from build123d import *

# Parameters (mm, degrees)
SKETCH1_R           = 3
BOSS_EXTRUDE2_DEPTH = 10
FILLET1_R           = 20
FILLET2_R           = 20
CUT_EXTRUDE1_START  = -10
CUT_EXTRUDE1_DEPTH  = 10
FILLET3_R           = 5
CUT_EXTRUDE4_START  = -10
CUT_EXTRUDE4_DEPTH  = 10


with BuildPart() as part:
    # Sketch1 → Boss-Extrude2 (new body)
    with BuildSketch(Plane.XY):
        with BuildLine():
            Line((-30, 15.770412854), (-30, 0))
            Line((-30, 0), (-17.5, -210))
            ThreePointArc((-17.5, -210), (0, -227.5), (17.5, -210))
            Line((17.5, -210), (30, 0))
            Line((30, 0), (30, 15.770412854))
            Line((30, 15.770412854), (-30, 15.770412854))
        make_face()
        with Locations((-15, 0)):
            Circle(SKETCH1_R, mode=Mode.SUBTRACT)
        with Locations((15, 0)):
            Circle(SKETCH1_R, mode=Mode.SUBTRACT)
        Polygon((0, -205), (6, -205), (6, -215), (-6, -215), (-6, -205), align=None, mode=Mode.SUBTRACT)
    extrude(amount=BOSS_EXTRUDE2_DEPTH)

    # Fillet1
    fillet1_edges = [part.edges().sort_by_distance(p)[0] for p in [
        (-30, 15.770412854, 5),
    ]]
    fillet(fillet1_edges, radius=FILLET1_R)

    # Fillet2
    fillet2_edges = [part.edges().sort_by_distance(p)[0] for p in [
        (30, 15.770412854, 5),
    ]]
    fillet(fillet2_edges, radius=FILLET2_R)

    # Sketch4 → Cut-Extrude1 (cut)
    with BuildSketch(Plane.XY.offset(10).offset(CUT_EXTRUDE1_START)):
        Polygon((-15.651797422, -15), (0.190220551, -102.160979768), (15.643622882, -15), (15, -15), align=None)
        Polygon((-22.473027071, -25.6531452), (-13.367328465, -178.628881795), (-4.134156204, -126.551525408), align=None)
        Polygon((22.230419841, -27.161313899), (4.615986353, -126.511039477), (13.430162671, -175.005634359), align=None)
        with BuildLine():
            Line((0.291609598, -150.901585116), (-7.372445375, -194.128735111))
            ThreePointArc((-7.372445375, -194.128735111), (0.476576628, -192.506490497), (8.225632191, -194.553674383))
            Line((8.225632191, -194.553674383), (0.291609598, -150.901585116))
        make_face()
    extrude(amount=CUT_EXTRUDE1_DEPTH, mode=Mode.SUBTRACT)

    # Fillet3
    fillet3_edges = [part.edges().sort_by_distance(p)[0] for p in [
        (8.225632191, -194.553674383, 5),
        (-7.372445375, -194.128735111, 5),
        (-15.651797422, -15, 5),
        (15.643622882, -15, 5),
    ]]
    fillet(fillet3_edges, radius=FILLET3_R)

    # Sketch5 → Cut-Extrude4 (cut)
    with BuildSketch(Plane.XY.offset(10).offset(CUT_EXTRUDE4_START)):
        with BuildLine():
            Line((29.260488635, 0), (18, 0))
            ThreePointArc((18, 0), (17.738612788, -1.224744871), (17, -2.236067977))
            Line((17, -2.236067977), (17, -18))
            Line((17, -18), (28.928571429, -18))
            Line((28.928571429, -18), (29.677502384, -5.417959945))
            ThreePointArc((29.677502384, -5.417959945), (29.653859351, -2.694751229), (29.260488635, 0))
        make_face()
        with BuildLine():
            ThreePointArc((17, 2.236067977), (17.738612788, 1.224744871), (18, 0))
            Line((18, 0), (29.260488635, 0))
            ThreePointArc((29.260488635, 0), (24.938968919, 8.738256866), (17, 14.39559177))
            Line((17, 14.39559177), (17, 2.236067977))
        make_face()
    extrude(amount=CUT_EXTRUDE4_DEPTH, mode=Mode.SUBTRACT)


solid = part.part
Build history of the part. All positions in model axes, mm. A direction names the side the tool comes from. Coordinates: 2 decimals unless noted, no trailing zeros. Write each loop counter-clockwise with the first axis right and the second up, starting at its lowest first coordinate (ties: lowest second). Pieces come first, ordered by that corner, then holes.
(1) Cut at B-B on y = -71.5. List the corners of the cut face in (x, z), and give its area (3 significant figures).
(2) Cut at C-C on z = 4.5. State how many separate pieces and enclosed holes the cut face has, and give its area (3 significant figures).
(3) Mould opens along Y. For faces 1 (the flat face through (7.295, -62.086, 4.93)), 2 (the cylindrical face through (-0.385, -227.496, 4.93)), 3 (the flat face through (-1, -104, 10)) say: pulls with the +Y half, pulls with the -Y half, needs draft (parallel to the pull), parting line crosses it, or undercut.
(4) Drill centre lines: line 1 (X direction, y = -43.5, z = 3.75); line 2 (X direction, y = -173, z = 4.75); line 3 (X direction, y = -145, z = 2.5). Where is each one in solid material? Low to high.
(5) Pin check, flat tips, straight feed: pin 1 Ø5 at (y, z) = (-209, 5) entering from +X; pin 2 Ø2 at (y, z) = (-190.5, 4) entering from +X; pin 3 Ø1 at (y, z) = (-15, 6) entering from +X. Stop position of each tip, or through.
(6) 3-axis set-ups, long thin cutter, end or side, ignore diameter. For faces 4 (the flat face through (-1, -104, 0)), 5 (the cylindrical face through (13.55, -16.835, 5.07)): which of +Z, -Z, +X, -X, +Y, -Y reach the whole face in a straight line?
(7) Cut at A-A on y = -117.5. List the corners of the cut face in (x, z), and give its area (3 significant figures).
Working result:
1. outline: (-25.74, 0) - (-19.74, 0) - (-19.74, 10) - (-25.74, 10) - close; (-14.14, 0) - (-5.38, 0) - (-5.38, 10) - (-14.14, 10) - close; (5.63, 0) - (14.37, 0) - (14.37, 10) - (5.63, 10) - close; (19.59, 0) - (25.74, 0) - (25.74, 10) - (19.59, 10) - close
1. area: 297 mm2
2. separate pieces: 1
2. enclosed holes: 6
2. area: 7,250 mm2
3. face 1: undercut
3. face 2: pulls with the -Y half
3. face 3: needs draft
4. line 1: x = -27.41 to -21.41, -19.23 to -10.47, 10.59 to 19.33, 21.26 to 27.41
4. line 2: x = -19.7 to -13.7, -12.37 to -3.63, 4.31 to 13.07, 13.55 to 19.7
4. line 3: x = -21.37 to -15.37, -7.41 to 7.98, 15.22 to 21.37
5. pin 1: stops at x = 17.71
5. pin 2: stops at x = 18.72
5. pin 3: stops at x = 17
6. face 4: -Z, +X, -X, +Y, -Y
6. face 5: +Z, -Z
7. outline: (-23.01, 0) - (-17.01, 0) - (-17.01, 10) - (-23.01, 10) - close; (-5.78, 0) - (6.21, 0) - (6.21, 10) - (-5.78, 10) - close; (16.85, 0) - (23.01, 0) - (23.01, 10) - (16.85, 10) - close
7. area: 241 mm2
